from build123d import *

# Parameters (mm, degrees)
ESQUISSE2_R             = 1.5
ENL_V_MAT_EXTRU_1_DEPTH = 7
ENL_V_MAT_EXTRU_2_REACH = 33
ESQUISSE3_R             = 1.5


with BuildPart() as part:
    # Esquisse1 → Révolution1 (revolve)
    with BuildSketch(Plane.XY):
        Polygon((0, 4), (-18, 4), (-18, 22), (-12, 22), (-12, 9), (-3, 9), (-3, 7.5), (0, 7.5), align=None)
    revolve(axis=Axis((0, 0, 0), (-1, 0, 0)))

    # Esquisse2 → Enlèv. mat.-Extru.1 (cut, through all)
    with BuildSketch(Plane(origin=(-12, 0, 0), x_dir=(0, 0, -1), z_dir=(1, 0, 0))):
        with Locations((0, 16)):
            Circle(ESQUISSE2_R)
        with Locations((13.856406461, -8)):
            Circle(ESQUISSE2_R)
        with Locations((-13.856406461, -8)):
            Circle(ESQUISSE2_R)
    extrude(amount=-ENL_V_MAT_EXTRU_1_DEPTH, mode=Mode.SUBTRACT)

    # Esquisse3 → Enlèv. mat.-Extru.2 (cut, up to next)
    with BuildSketch(Plane(origin=(0, 9, 0), x_dir=(1, 0, 0), z_dir=(0, 1, 0)), mode=Mode.PRIVATE) as enl_v_mat_extru_2_sk1:
        with Locations((-7.5, 0)):
            Circle(ESQUISSE3_R)
    enl_v_mat_extru_2_tool1 = extrude(enl_v_mat_extru_2_sk1.sketch, amount=-ENL_V_MAT_EXTRU_2_REACH, mode=Mode.PRIVATE) & part.part
    add(enl_v_mat_extru_2_tool1.solids().sort_by_distance((-7.5, 9, 0))[0], mode=Mode.SUBTRACT)


solid = part.part
Part model, mm, in its own coordinate system. A direction names the side the tool comes from. Coordinates: 2 decimals unless noted, no trailing zeros. Order: outer loops, then holes, each group sorted by start corner. A loop starts at its lowest first (then second) coordinate and runs counter-clockwise, first axis right, second up. Notation, with made-up numbers: M 18.5,71.25 L 49.5,71.25 A23 cw 49.5,102.25 Z; hole C 74.5,-22 d2. An arc over 180 degrees is marked long. Use a Markdown table: item, result.
(1) Flat gauge pins, fed straight in: pin 1 (2.5 mm diameter, centred on x = -7.5, z = 0, fed in from -Y); pin 2 (10 mm diameter, centred on y = -12.5, z = -14.5, fed in from +X); pin 3 (1.5 mm diameter, centred on x = -13.5, y = -17.5, fed in from -Z). Where does each tip first touch, or does it go through?
A:
| item | result |
|---|---|
| pin 1 | stops at y = -9 |
| pin 2 | stops at x = -12 |
| pin 3 | stops at z = -14.26 |
(2) Cut at B-B on z = 0. Write the cut outline in (x, y), then the cut area to 3 significant figures.
A:
| item | result |
|---|---|
| outline | M -18,-22 L -12,-22 L -12,-9 L -3,-9 L -3,-7.5 L 0,-7.5 L 0,-4 L -18,-4 Z; M -18,4 L -9,4 L -9,9 L -12,9 L -12,14.5 L -18,14.5 Z; M -18,17.5 L -12,17.5 L -12,22 L -18,22 Z; M -6,4 L 0,4 L 0,7.5 L -3,7.5 L -3,9 L -6,9 Z |
| area | 294 mm^2 |
(3) Cut at D-D on z = -5. Write the cut outline in (x, y), then the cut area to 3 significant figures.
A:
| item | result |
|---|---|
| outline | M -18,-21.42 L -12,-21.42 L -12,-7.48 L -3,-7.48 L -3,-5.59 L 0,-5.59 L 0,5.59 L -3,5.59 L -3,7.48 L -12,7.48 L -12,21.42 L -18,21.42 Z |
| area | 425 mm^2 |
(4) Cut at A-A on y = 0. Write the cut outline in (x, z).
A:
| item | result |
|---|---|
| outline | M -18,-22 L -12,-22 L -12,-9 L -3,-9 L -3,-7.5 L 0,-7.5 L 0,-4 L -18,-4 Z; M -18,4 L 0,4 L 0,7.5 L -3,7.5 L -3,9 L -12,9 L -12,22 L -18,22 Z |
(5) Tool access for faces 5 (the cylindrical face through (-14.96, 17.01, 1.11)), 6 (the cylindrical face through (-7.437, -1.172, -8.923)), 7 (the cylindrical face through (-9, 6, 0)): list every direction of +Z, -Z, +X, -X, +Y, -Y with a clear straight run to the whole face (end or side of a thin tool).
A:
| item | result |
|---|---|
| face 5 | +X, -X |
| face 6 | +X |
| face 7 | +Y |
(6) Pull direction Z, two halves, no side cores. Call faces 1 (the cylindrical face through (-14.96, -8.91, 15.05)), 2 (the flat face through (0, 3, 3)), 3 (the cylindrical face through (-1.479, -7.493, -0.33)), 4 (the cylindrical face through (-14.958, -9.464, -13.531)): released by +Z, released by -Z, zero draft, split by the parting line, or undercut.
A:
| item | result |
|---|---|
| face 1 | undercut |
| face 2 | zero draft |
| face 3 | split by the parting line |
| face 4 | undercut |
(7) Cut at C-C on x = -16.5. Write the cut outline in (y, z), then the cut area to 3 significant figures.
A:
| item | result |
|---|---|
| outline | C 0,0 d44; hole C -8,-13.86 d3; hole C -8,13.86 d3; hole C 0,0 d8; hole C 16,0 d3 |
| area | 1,450 mm^2 |
(8) Probe L1, parallel to Y at x = -13.3, z = 0; L2, parallel to Y at x = -5.75, z = 0; L3, parallel to X at y = 5, z = 0. List the from-to ranges inside material, lowest first.
A:
| item | result |
|---|---|
| L1 | y = -22 to -4, 4 to 14.5, 17.5 to 22 |
| L2 | y = -9 to -4, 4 to 9 |
| L3 | x = -18 to -9, -6 to 0 |
